Read the model definition and answer for the solid it produces. Units are mm, in the model's axes. Face numbers are marked on the shaded views. Coordinates: 2 decimals unless noted, no trailing zeros. Order: outer loops, then holes, each group sorted by start corner. A loop starts at its lowest first (then second) coordinate and runs counter-clockwise, first axis right, second up. Notation, with made-up numbers: M 73.5,65.5 L 89.5,65.5 A22 cw 89.5,74.5 Z; hole C -40,49.25 d5. An arc over 180 degrees is marked long. Write each question's results on one line, items separated by ' | '.
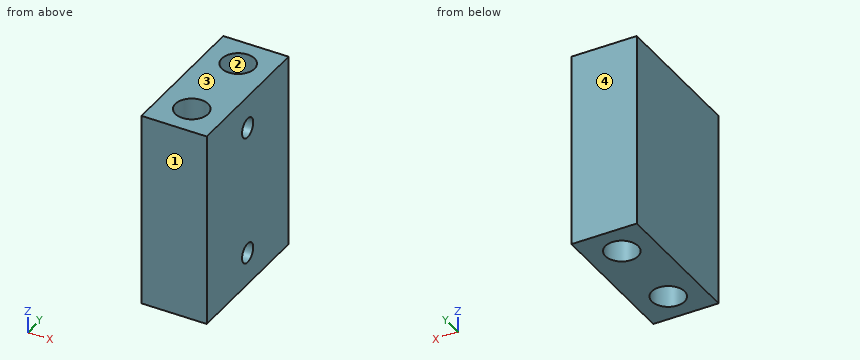
```python
from build123d import *

# Parameters (mm, degrees)
F0_W     = 20
F0_H     = 44
F0_R     = 5
F1_DEPTH = 60
F2_R     = 3
F3_DEPTH = 10


with BuildPart() as f1:
    # F0 (on Top) → F1 (new body)
    with BuildSketch(Plane.XY):
        Rectangle(F0_W, F0_H)
        with Locations((0, -12.5)):
            Circle(F0_R, mode=Mode.SUBTRACT)
        with Locations((0, 12.5)):
            Circle(F0_R, mode=Mode.SUBTRACT)
    extrude(amount=F1_DEPTH)

    # F2 (on face) → F3 (cut)
    with BuildSketch(Plane.YZ.offset(10)):
        with Locations((0, 50)):
            Circle(F2_R)
        with Locations((0, 10)):
            Circle(F2_R)
    extrude(amount=-F3_DEPTH, mode=Mode.SUBTRACT)


solid = f1.part
```
(1) The part is cut by section B-B, the plane y = 12.5. Write down the section's boundary in (x, z).
Conclusion:
outline: M -10,0 L -5,0 L -5,60 L -10,60 Z; M 5,0 L 10,0 L 10,60 L 5,60 Z
(2) The part is cut by section C-C, the plane x = -0.75. Write down the section's boundary in (y, z), then the cut area to 3 significant figures.
Conclusion:
outline: M -22,0 L -17.44,0 L -17.44,60 L -22,60 Z; M -7.56,0 L 7.56,0 L 7.56,60 L -7.56,60 Z; M 17.44,0 L 22,0 L 22,60 L 17.44,60 Z | area: 1,450 mm²
(3) The part is cut by section D-D, the plane y = 0. Write down the section's boundary in (x, z), then the cut area to 3 significant figures.
Conclusion:
outline: M -10,0 L 10,0 L 10,7 L 0,7 L 0,13 L 10,13 L 10,47 L 0,47 L 0,53 L 10,53 L 10,60 L -10,60 Z | area: 1,080 mm²
(4) The mould has two halves that part along Y. Classify the marked faces 1, 2, 3 and 4: pulls with the +Y half, pulls with the -Y half, needs draft (parallel to the pull), parting line crosses it, or undercut.
Conclusion:
face 1: pulls with the -Y half | face 2: undercut | face 3: needs draft | face 4: pulls with the +Y half
(5) Straight lines are drawn through the part: line 1 (Z direction, x = 5.5, y = 0); line 2 (Y direction, x = 0, z = 24); line 3 (Y direction, x = 1.75, z = 9). For each, find the intervals that lie inside material, in ascending order.
Conclusion:
line 1: 0 to 7, 13 to 47, 53 to 60 | line 2: -22 to -17.5, -7.5 to 7.5, 17.5 to 22 | line 3: -22 to -17.18, -7.82 to -2.83, 2.83 to 7.82, 17.18 to 22
(6) The part is cut by section A-A, the plane x = 2.75. Write down the section's boundary in (y, z), then the cut area to 3 significant figures.
Conclusion:
outline: M -22,0 L -16.68,0 L -16.68,60 L -22,60 Z; M -8.32,0 L 8.32,0 L 8.32,60 L -8.32,60 Z; M 16.68,0 L 22,0 L 22,60 L 16.68,60 Z; hole C 0,10 d6; hole C 0,50 d6 | area: 1,580 mm²
(7) Given pin 1 (1.8 mm diameter, centred on y = 0.5, z = 9.5, fed in from +X), flat-ended and moving along its own axis, determine where the tip first touches the part or whether it passes through.
Conclusion:
pin 1: x = 0
